Part model, mm, in its own coordinate system. Face numbers are marked on the shaded views. A direction names the side the tool comes from. Round coordinates to 2 decimals unless told otherwise and drop trailing zeros. Order: outer loops, then holes, each group sorted by start corner. A loop starts at its lowest first (then second) coordinate and runs counter-clockwise, first axis right, second up. Notation, with made-up numbers: (-40, -14.75) - (-3, -14.75) arc R23 ccw to (-3, 13.25) - close; hole circle Ø8 at (-10.75, -35.75). An arc over 180 degrees is marked (long way). Return JSON: item names as keys, results as strings. Group by question number.
Item 1: Probe probe 1 along Y at (x, z) = (0, -5.5); probe 2 along Y at (x, z) = (-1.25, -7.75); probe 3 along X at (y, z) = (-1.5, -2.75). List the from-to ranges inside material, lowest first.
Item 2: Saw through at B-B on y = 3.5. List the corners of the cut face in (x, z), and give its area (3 significant figures).
Item 3: Tool access for the marked faces 4 and 5: list every direction of +Z, -Z, +X, -X, +Y, -Y with a clear straight run to the whole face (end or side of a thin tool).
Item 4: Drop flat-ended pins along their axis: pin 1 (1.5 mm diameter, centred on y = 3.5, z = 1, fed in from +X); pin 2 (1 mm diameter, centred on y = 1.5, z = -2.5, fed in from +X); pin 3 (3 mm diameter, centred on y = 2, z = -0.5, fed in from +X). Give the stop position or say it passes through.
Item 5: Saw through at D-D on x = 3. List the corners of the cut face in (y, z), and give its area (3 significant figures).
Item 6: Saw through at C-C on z = -1.5. List the corners of the cut face in (x, y).
Item 7: Saw through at A-A on x = 0. List the corners of the cut face in (y, z).
Item 8: Two-plate mould, pull along Z, no slides. Class the marked faces 1, 2 and 3: released by +Z, released by -Z, zero draft, split by the parting line, or undercut.
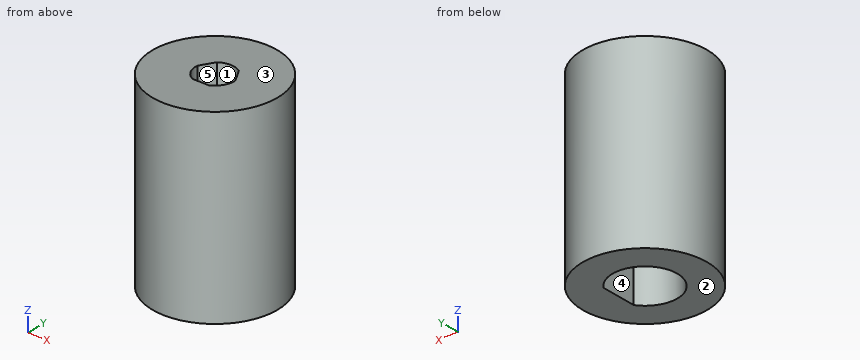
Autodesk Inventor part; units mm, degrees
ref_plane "YZ Plane" through (0, 0, 0) normal (1, 0, 0) x (0, 1, 0)
ref_plane "XZ Plane" through (0, 0, 0) normal (0, 1, 0) x (-1, 0, 0)
ref_plane "XY Plane" through (0, 0, 0) normal (0, 0, 1) x (1, 0, 0)
sketch "Sketch1" plane through (0, 0, 0) normal (0, 0, 1) x (1, 0, 0)
  circle A0 centre (0, 0) radius 2.5
  circle A1 centre (0, 0) radius 2.6
  line L0 (-1.3981, 2.1921) -> (1.3981, 2.1921)
  circle A2 centre (0, 0) radius 5
  dimension "d0" = 0.1
  dimension "d1" = 10
extrude "Extrusion1" add sketch "Sketch1" against normal blind 10
sketch "Sketch2" plane through (0, 0, 0) normal (0, 0, 1) x (1, 0, 0)
  circle A0 centre (0, 0) radius 1.4 construction
  line L0 (0.6514, -1.4) -> (-0.6514, -1.4)
  line L1 (1.5381, 0.1359) -> (0.8867, 1.2641)
  line L2 (-0.8867, 1.2641) -> (-1.5381, 0.1359)
  arc A1 (0.6514, -1.4) -> (1.5381, 0.1359) centre (0, 0) ccw
  arc A2 (-1.5381, 0.1359) -> (-0.6514, -1.4) centre (0, 0) ccw
  arc A3 (0.8867, 1.2641) -> (-0.8867, 1.2641) centre (0, 0) ccw
  circle A4 centre (0, 0) radius 5
  dimension "d4" = 2.8
  dimension "d9" = 60
  dimension "d10" = 60
extrude "Extrusion2" add sketch "Sketch2" along normal blind 5
sketch "Sketch3" plane through (0, 0, -10) normal (0, 0, -1) x (-1, 0, 0)
  line L0 (-2.1363, -1.482) -> (-2.1363, 1.482)
  circle A0 centre (0, 0) radius 2.6
extrude "Extrusion3" add sketch "Sketch3" against normal up to surface (10 mm away) contours A0 L0 picked at (-2.2341, 0.3085)
properties part number "OPENTRONS_Autofocus_clutch_Nema"
Filled in:
{
 "1": {"probe 1": "y = -5 to -2.6, 2.6 to 5", "probe 2": "y = -4.84 to -2.28, 2.28 to 4.84", "probe 3": "x = -4.77 to -2.12, 2.12 to 4.77"},
 "2": {"outline": "(-3.57, -10) - (3.57, -10) - (3.57, 5) - (-3.57, 5) - close", "area": "107 mm^2"},
 "3": {"face 4": "-Z", "face 5": "+Z, -Z"},
 "4": {"pin 1": "stops at x = 4.18", "pin 2": "stops at x = 4.9", "pin 3": "stops at x = 4.97"},
 "5": {"outline": "(-4, -10) - (4, -10) - (4, 5) - (-4, 5) - close", "area": "120 mm^2"},
 "6": {"outline": "circle Ø10 at (0, 0); hole (2.14, -1.48) - (2.14, 1.48) arc R2.6 ccw (long way) to start"},
 "7": {"outline": "(-5, -10) - (-2.6, -10) - (-2.6, 0) - (-1.4, 0) - (-1.4, 5) - (-5, 5) - close; (1.54, 0) - (2.6, 0) - (2.6, -10) - (5, -10) - (5, 5) - (1.54, 5) - close"},
 "8": {"face 1": "zero draft", "face 2": "released by -Z", "face 3": "released by +Z"}
}
